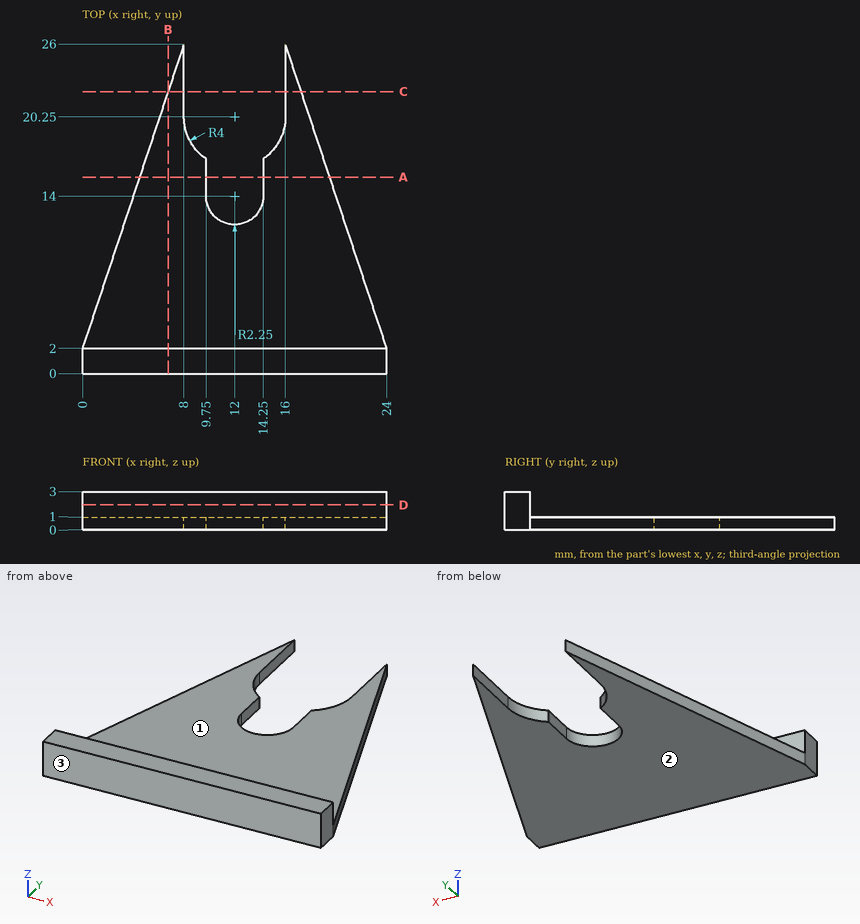
Answer from the drawing. Dimensions are ordinates in mm from the lowest x, y and z of the part. Round coordinates to 2 decimals unless told otherwise and drop trailing zeros. Loops run counter-clockwise (first coordinate to the right, second up) from the corner with the lowest first, then second, coordinate; pieces in that order, holes last. Notation, with made-up numbers: M 28.25,-3.5 L 66.25,-3.5 A16 ccw 66.25,16.5 Z; hole C 82.25,47 d1. An arc over 180 degrees is marked long. One line per question, with ' | ' between items. Start each with the question number.
(1) A cutting plane is placed at D-D on z = 1.95. Write down the section's boundary in (x, y).
(2) Flat-ended cylindrical pins translate along their axes: pin 1 Ø0.8 at (y, z) = (16, 0.5) entering from +X; pin 2 Ø0.5 at (y, z) = (15.5, 0.5) entering from -X; pin 3 Ø1 at (x, z) = (7, 2) entering from +Y. Find the tip coordinate at first contact, or state that the pin passes through.
(3) For a pull along Z with two mould halves and no side action, classify the marked faces 1, 2 and 3 as released by +Z, released by -Z, zero draft, split by the parting line, or undercut.
(4) A cutting plane is placed at B-B on x = 6.75. Write down the section's boundary in (y, z), plus the area to 4 significant figures.
(5) Find the intervals of material crossed by line 1 (Y direction, x = 21.5, z = 1.4); line 2 (Z direction, x = 18, y = 11.75); line 3 (X direction, y = 15, z = 0.35), in increasing order.
(6) A cutting plane is placed at A-A on y = 15.5. Write down the section's boundary in (x, z).
(7) A cutting plane is placed at C-C on y = 22.25. Write down the section's boundary in (x, z).
Geometry check:
1) outline: M 0,0 L 24,0 L 24,2 L 0,2 Z
2) pin 1: stops at x = 19.47 | pin 2: stops at x = 4.42 | pin 3: stops at y = 2
3) face 1: released by +Z | face 2: released by -Z | face 3: zero draft
4) outline: M 0,0 L 22.25,0 L 22.25,1 L 2,1 L 2,3 L 0,3 Z | area: 26.25 mm²
5) line 1: y = 0 to 2 | line 2: z = 0 to 1 | line 3: x = 4.33 to 9.75, 14.25 to 19.67
6) outline: M 4.5,0 L 9.75,0 L 9.75,1 L 4.5,1 Z; M 14.25,0 L 19.5,0 L 19.5,1 L 14.25,1 Z
7) outline: M 6.75,0 L 8,0 L 8,1 L 6.75,1 Z; M 16,0 L 17.25,0 L 17.25,1 L 16,1 Z
